from build123d import *

# Parameters (mm, degrees)
SKETCH_1_R      = 5.5
SKETCH_1_R_2    = 2.5
EXTRUDE_1_DEPTH = 12.5
EXTRUDE_2_DEPTH = 4.5


with BuildPart() as part:
    # 草图1 → 凸台-拉伸1 (new body)
    with BuildSketch(Plane.XY):
        Circle(SKETCH_1_R)
        Circle(SKETCH_1_R_2, mode=Mode.SUBTRACT)
    extrude(amount=EXTRUDE_1_DEPTH)

    # 草图2 → 凸台-拉伸2 (add)
    with BuildSketch(Plane.XY.offset(12.5)):
        Polygon((-3.5, 6.062177826), (3.5, 6.062177826), (7, 0), (3.5, -6.062177826), (-3.5, -6.062177826), (-7, 0), align=None)
    extrude(amount=EXTRUDE_2_DEPTH)


solid = part.part
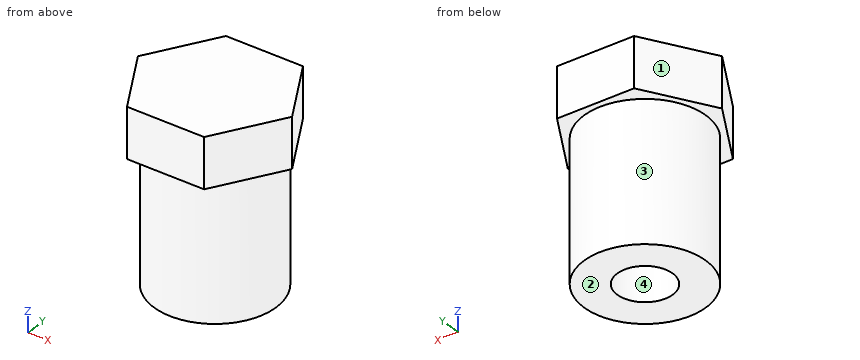
The listing builds one solid part. Answer for the finished solid, in the listing's coordinates (mm). Face numbers are marked on the shaded views. Coordinates: 2 decimals unless noted, no trailing zeros. Write each loop counter-clockwise with the first axis right and the second up, starting at its lowest first coordinate (ties: lowest second). Pieces come first, ordered by that corner, then holes. Notation, with made-up numbers: M 37.5,40.25 L 72.5,40.25 A9 cw 72.5,55.25 Z; hole C 1.5,-28 d1. An arc over 180 degrees is marked long. Write each question's results on one line, items separated by ' | '.
Item 1: The part is cut by section C-C on y = -1.75. Determine the outline of the cut face in (x, z).
Answer below:
outline: M -5.99,12.5 L -5.21,12.5 L -5.21,0 L -1.79,0 L -1.79,12.5 L 1.79,12.5 L 1.79,0 L 5.21,0 L 5.21,12.5 L 5.99,12.5 L 5.99,17 L -5.99,17 Z
Item 2: For a pull along X with two mould halves and no side action, classify the marked faces 1, 2, 3 and 4 as released by +X, released by -X, zero draft, split by the parting line, or undercut.
Answer below:
face 1: released by -X | face 2: zero draft | face 3: split by the parting line | face 4: undercut
Item 3: The part is cut by section A-A on z = 11.5. Determine the outline of the cut face in (x, y).
Answer below:
outline: C 0,0 d11; hole C 0,0 d5
Item 4: The part is cut by section B-B on x = 0. Determine the outline of the cut face in (y, z).
Answer below:
outline: M -6.06,12.5 L -5.5,12.5 L -5.5,0 L -2.5,0 L -2.5,12.5 L 2.5,12.5 L 2.5,0 L 5.5,0 L 5.5,12.5 L 6.06,12.5 L 6.06,17 L -6.06,17 Z
Item 5: Given P1, Ø2.5, axis at x = -0.5, y = -0.5, coming from the -Z side; P2, Ø6, axis at y = 5, z = 7.5, coming from the -X side; P3, Ø6, axis at x = 2.5, z = 1.5, coming from the -Y side, each flat-ended and moving along its own axis, determine where each tip first touches the part or whether it passes through.
Answer below:
P1: z = 12.5 | P2: x = -5.12 | P3: y = -5.5
Item 6: Consider probe 1 along Y at (x, z) = (0, 4.5); probe 2 along Y at (x, z) = (-0.75, 6.5); probe 3 along X at (y, z) = (1.25, 11). Determine where each line is inside the solid, lowest interval first. Write a range as [from, to].
Answer below:
probe 1: [-5.5, -2.5], [2.5, 5.5] | probe 2: [-5.45, -2.38], [2.38, 5.45] | probe 3: [-5.36, -2.17], [2.17, 5.36]
Item 7: The part is cut by section D-D on x = 5.25. Determine the outline of the cut face in (y, z), and give its area (3 significant figures).
Answer below:
outline: M -3.03,12.5 L -1.64,12.5 L -1.64,0 L 1.64,0 L 1.64,12.5 L 3.03,12.5 L 3.03,17 L -3.03,17 Z | area: 68.3 mm2
